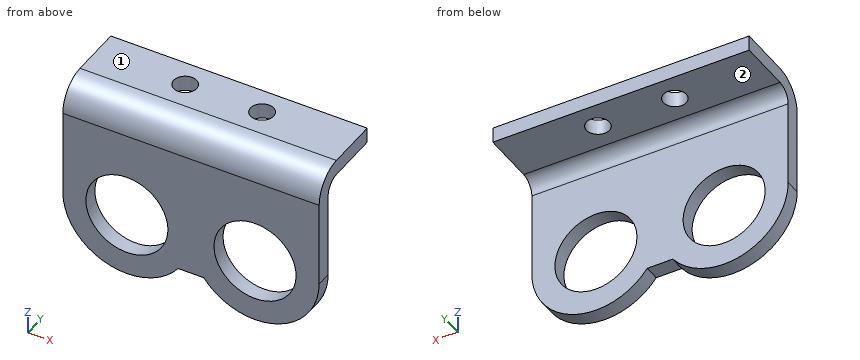
```python
from build123d import *

# Parameters (mm, degrees)
SKETCH_1_R                       = 8
SM_BASE_FLANGE_1_DEPTH           = 3
SM_EDGE_FLANGE_1_STRIP_W         = 17.4732
SM_EDGE_FLANGE_1_STRIP_H         = 3
SM_EDGE_FLANGE_1_STRIP_CUT_DEPTH = 50
SM_EDGE_FLANGE_1_DEPTH           = 50
SKETCH_9_R                       = 2.25
CUT_EXTRUDE_1_DEPTH              = 10


# Sheet-metal steps are written as plain solids
with BuildPart() as part:
    # Sketch 1 → 基体-法兰1 (new body)
    with BuildSketch(Plane(origin=(0, 0, 0), x_dir=(1, 0, 0), z_dir=(0, 1, 0))):
        with BuildLine():
            Line((-25, 22.5), (-25, 0))
            Line((-25, 0), (25, 0))
            Line((25, 0), (25, 22.5))
            ThreePointArc((25, 22.5), (16.452847075, 34.358541226), (2.5, 30))
            Line((2.5, 30), (-2.5, 30))
            ThreePointArc((-2.5, 30), (-16.452847075, 34.358541226), (-25, 22.5))
        make_face()
        with Locations(Location((-12.5, 22.5, 0), (0, 0, 270))):
            Circle(SKETCH_1_R, mode=Mode.SUBTRACT)
        with Locations(Location((12.5, 22.5, 0), (0, 0, 90))):
            Circle(SKETCH_1_R, mode=Mode.SUBTRACT)
    extrude(amount=-SM_BASE_FLANGE_1_DEPTH)

    # 边线-法兰1 strip (across the edge) → 边线-法兰1 strip cut (cut)
    with BuildSketch(Plane(origin=(-25, 0, 0), x_dir=(0, 0, -1), z_dir=(1, 0, 0))):
        with Locations((-3, -1.5)):
            Rectangle(SM_EDGE_FLANGE_1_STRIP_W, SM_EDGE_FLANGE_1_STRIP_H)
    extrude(amount=SM_EDGE_FLANGE_1_STRIP_CUT_DEPTH, mode=Mode.SUBTRACT)

    # 边线-法兰1 section (across the edge) → 边线-法兰1 (add)
    with BuildSketch(Plane(origin=(-25, 0, 0), x_dir=(0, 0, -1), z_dir=(1, 0, 0))):
        with BuildLine():
            Line((0, 2.7366), (0, 13))
            Line((0, 13), (3, 13))
            Line((3, 13), (3, 2.7366))
            ThreePointArc((3, 2.7366), (3.801531583, 0.801531583), (5.7366, 0))
            Line((5.7366, 0), (5.7366, -3))
            ThreePointArc((5.7366, -3), (1.680211239, -1.319788761), (0, 2.7366))
        make_face()
    extrude(amount=SM_EDGE_FLANGE_1_DEPTH)

    # 草图9 → 切除-拉伸1 (cut)
    with BuildSketch(Plane.XY):
        with Locations((7.5, 7.8683)):
            Circle(SKETCH_9_R)
        with Locations(Location((-7.5, 7.8683, 0), (0, 0, 270))):
            Circle(SKETCH_9_R)
    extrude(amount=-CUT_EXTRUDE_1_DEPTH, mode=Mode.SUBTRACT)


solid = part.part
```
The listing builds one solid part. Answer for the finished solid, in the listing's coordinates (mm). Face numbers are marked on the shaded views. A direction names the side the tool comes from. Give positions to 0.01 mm unless a question says otherwise; leave off trailing zeros. Order: outer loops, then holes, each group sorted by start corner. A loop starts at its lowest first (then second) coordinate and runs counter-clockwise, first axis right, second up. Notation, with made-up numbers: (46, -3) -> (68, -3) arc R20 ccw to (68, 28) -> close; hole circle Ø5 at (44.25, 77.25). An arc over 180 degrees is marked (long way). Answer as CSV lines item,"result". Start each with the question number.
Q1. A cutting plane is placed at D-D (x = -7.5). Determine the outline of the cut face in (y, z) (3 decimals).
Q2. A cutting plane is placed at C-C (z = -28). Determine the outline of the cut face in (x, y), then the cut area to 3 significant figures.
Q3. Find the intervals of material crossed by L1, parallel to X at y = -1.5, z = -22.5; L2, parallel to Z at x = 18, y = 3; L3, parallel to Z at x = 17.5, y = -0.25 (3 decimals), in increasing order.
Q4. Which of the six approach directions +Z, -Z, +X, -X, +Y, -Y give full straight-line access (tool end or side, diameter ignored) to the marked faces 1 and 2?
Q5. A cutting plane is placed at B-B (y = 6.5). Determine the outline of the cut face in (x, z), then the cut area to 3 significant figures.
Q6. Given pin 1 (3.5 mm diameter, centred on x = 0, y = -2, fed in from -Z); pin 2 (3 mm diameter, centred on x = -3.5, y = 10.5, fed in from -Z); pin 3 (1 mm diameter, centred on x = -3.5, y = 0, fed in from +Z), each flat-ended and moving along its own axis, determine where each tip first touches the part or whether it passes through.
Q7. A cutting plane is placed at A-A (x = -12.5). Determine the outline of the cut face in (y, z).
Results found:
1,outline,"(-3, -33.956) -> (0, -33.956) -> (0, -28.745) -> (-3, -28.745) -> close; (-3, -16.255) -> (0, -16.255) -> (0, -5.737) arc R2.737 cw to (2.737, -3) -> (5.618, -3) -> (5.618, 0) -> (2.737, 0) arc R5.737 ccw to (-3, -5.737) -> close; (10.118, -3) -> (13, -3) -> (13, 0) -> (10.118, 0) -> close"
2,outline,"(-23.72, -3) -> (-18.31, -3) -> (-18.31, 0) -> (-23.72, 0) -> close; (-6.69, -3) -> (6.69, -3) -> (6.69, 0) -> (-6.69, 0) -> close; (18.31, -3) -> (23.72, -3) -> (23.72, 0) -> (18.31, 0) -> close"
2,area,"72.6 mm2"
3,L1,"-25 to -20.5, -4.5 to 4.5, 20.5 to 25"
3,L2,"-3 to 0"
3,L3,"-33.956 to -28.745, -16.255 to -0.839"
4,face 1,"+Z, +X, -X, +Y, -Y"
4,face 2,"-Z, +X, -X, +Y"
5,outline,"(-25, -3) -> (-9.29, -3) -> (-9.29, 0) -> (-25, 0) -> close; (-5.71, -3) -> (5.71, -3) -> (5.71, 0) -> (-5.71, 0) -> close; (9.29, -3) -> (25, -3) -> (25, 0) -> (9.29, 0) -> close"
5,area,"129 mm2"
6,pin 1,"z = -30"
6,pin 2,"z = -3"
6,pin 3,"z = -0.45"
7,outline,"(-3, -35) -> (0, -35) -> (0, -30.5) -> (-3, -30.5) -> close; (-3, -14.5) -> (0, -14.5) -> (0, -5.74) arc R2.74 cw to (2.74, -3) -> (13, -3) -> (13, 0) -> (2.74, 0) arc R5.74 ccw to (-3, -5.74) -> close"
